Autodesk Inventor part; units mm, degrees
ref_plane "YZ Plane" through (0, 0, 0) normal (1, 0, 0) x (0, 1, 0)
ref_plane "XZ Plane" through (0, 0, 0) normal (0, 1, 0) x (-1, 0, 0)
ref_plane "XY Plane" through (0, 0, 0) normal (0, 0, 1) x (1, 0, 0)
sketch "Sketch2" plane through (0, 0, 0) normal (0, 0, 1) x (1, 0, 0)
  line L0 (0, 12.7) -> (3.6703, 12.7)
  line L1 (0, 12.7) -> (-3.6703, 12.7)
  line L2 (0, 0) -> (3.6703, 0)
  line L3 (0, 0) -> (-3.6703, 0)
  line L4 (-3.6703, 0) -> (-7.3406, 6.35)
  line L5 (-7.3406, 6.35) -> (-3.6703, 12.7)
  line L6 (3.6703, 12.7) -> (7.3406, 6.35)
  line L7 (7.3406, 6.35) -> (3.6703, 0)
  line L8 (0, 0) -> (0, 6.35)
  circle A0 centre (0, 6.35) radius 8.255
  dimension "d11" = 6.35
  dimension "d12" = 16.51
extrude "Extrusion2" add sketch "Sketch2" along normal blind 6.223
sketch "Sketch3" plane through (0, 6.35, 6.223) normal (0, 0, 1) x (1, 0, 0)
  line L0 (-3.6703, -6.35) -> (-7.3406, 0)
  line L1 (-7.3406, 0) -> (-3.6703, 6.35)
  line L2 (-3.6703, 6.35) -> (3.6703, 6.35)
  line L3 (3.6703, 6.35) -> (7.3406, 0)
  line L4 (7.3406, 0) -> (3.6703, -6.35)
  line L5 (3.6703, -6.35) -> (-3.6703, -6.35)
  circle A0 centre (0, 0) radius 8.255
  point P0 (0, -6.35)
extrude "Extrusion3" add sketch "Sketch3" along normal blind 3.302
sketch "Sketch4" plane through (0, 6.35, 9.525) normal (0, 0, 1) x (1, 0, 0)
  line L0 (-7.3406, 0) -> (-3.6703, 6.35)
  line L1 (-3.6703, 6.35) -> (3.6703, 6.35)
  line L2 (3.6703, 6.35) -> (7.3406, 0)
  line L3 (7.3406, 0) -> (3.6703, -6.35)
  line L4 (3.6703, -6.35) -> (-3.6703, -6.35)
  line L5 (-3.6703, -6.35) -> (-7.3406, 0)
  circle A0 centre (0, 0) radius 8.255
  point P0 (0, -6.35)
extrude "Extrusion4" add sketch "Sketch4" along normal blind 6.5786
sketch "Sketch5" plane through (0, 6.35, 16.1036) normal (0, 0, 1) x (1, 0, 0)
  line L0 (-16.3467, 15.7745) -> (15.1254, 15.7745)
  line L1 (15.1254, 15.7745) -> (15.1254, -12.8793)
  line L2 (15.1254, -12.8793) -> (-16.3467, -12.8793)
  line L3 (-16.3467, -12.8793) -> (-16.3467, 15.7745)
  point P0 (0, -6.35)
extrude "Extrusion5" cut sketch "Sketch5" against normal blind 6.5786
sketch "Sketch8" plane through (0, 6.35, 9.525) normal (0, 0, 1) x (1, 0, 0)
  line L0 (-7.3406, 0) -> (-3.6703, -6.35)
  line L1 (-3.6703, 6.35) -> (-7.3406, 0)
  line L2 (3.6703, 6.35) -> (-3.6703, 6.35)
  line L3 (7.3406, 0) -> (3.6703, 6.35)
  line L4 (3.6703, -6.35) -> (7.3406, 0)
  line L5 (-3.6703, -6.35) -> (3.6703, -6.35)
  circle A0 centre (0, 0) radius 8.255
  point P0 (0, -6.35)
extrude "Extrusion7" add sketch "Sketch8" along normal blind 15.875
sketch "Sketch9" plane through (0, 6.35, 25.4) normal (0, 0, 1) x (1, 0, 0)
  line L0 (-7.3406, 0) -> (-3.6703, 6.35)
  line L1 (-3.6703, 6.35) -> (3.6703, 6.35)
  line L2 (3.6703, 6.35) -> (7.3406, 0)
  line L3 (7.3406, 0) -> (3.6703, -6.35)
  line L4 (3.6703, -6.35) -> (-3.6703, -6.35)
  line L5 (-3.6703, -6.35) -> (-7.3406, 0)
  circle A0 centre (0, 0) radius 8.255
  point P0 (0, -6.35)
extrude "Extrusion8" cut sketch "Sketch9" against normal blind 21.7424
sketch "Sketch10" plane through (0, 6.35, 3.6576) normal (0, 0, 1) x (1, 0, 0)
  line L0 (-7.3406, 0) -> (-3.6703, -6.35)
  line L1 (-3.6703, 6.35) -> (-7.3406, 0)
  line L2 (3.6703, 6.35) -> (-3.6703, 6.35)
  line L3 (7.3406, 0) -> (3.6703, 6.35)
  line L4 (3.6703, -6.35) -> (7.3406, 0)
  line L5 (-3.6703, -6.35) -> (3.6703, -6.35)
  circle A0 centre (0, 0) radius 8.255
  point P0 (0, -6.35)
extrude "Extrusion9" add sketch "Sketch10" along normal blind 9.1948
sketch "Sketch11" plane through (0, 6.35, 12.8524) normal (0, 0, 1) x (1, 0, 0)
  line L0 (-15.4934, 11.3446) -> (16.2643, 11.3446)
  line L1 (16.2643, 11.3446) -> (16.2643, -11.0726)
  line L2 (16.2643, -11.0726) -> (-15.4934, -11.0726)
  line L3 (-15.4934, -11.0726) -> (-15.4934, 11.3446)
  point P0 (0, -6.35)
extrude "Extrusion10" cut sketch "Sketch11" against normal blind 1.651
properties part number ".441Spacer"
The listing builds one solid part. Answer for the finished solid, in the listing's coordinates (mm). A direction names the side the tool comes from. Coordinates: 2 decimals unless noted, no trailing zeros. Loops run counter-clockwise (first coordinate to the right, second up) from the corner with the lowest first, then second, coordinate; pieces in that order, holes last. Notation, with made-up numbers: M -33.75,14 L 1.25,14 A34 cw 1.25,49 Z; hole C 86,76.5 d9. An arc over 180 degrees is marked long. Answer as a JSON object with one key per item and string values. Group by question number.
Item 1: Consider L1, parallel to X at y = 4.25, z = 10; L2, parallel to X at y = 3.5, z = 8; L3, parallel to Y at x = 3.75, z = 1.5. Determine where each line is inside the solid, lowest interval first.
Item 2: Section D-D (y = 13) is taken. Write down the section's boundary in (x, z), and give its area (3 significant figures).
Item 3: Section A-A (x = 0) is taken. Write down the section's boundary in (y, z) (3 decimals), and give its area (3 significant figures).
Item 4: Each of these flat-tipped pins is pushed along its axis until it touches: P1, Ø5, axis at y = 3.5, z = 10, coming from the +X side; P2, Ø5, axis at x = -4, z = 3, coming from the +Y side; P3, Ø4, axis at y = 9.5, z = 7, coming from the -X side. Where does it stop, or does it pass through?
Item 5: Section C-C (y = 8.75) is taken. Write down the section's boundary in (x, z).
Item 6: Section B-B (z = 3) is taken. Write down the section's boundary in (x, y) (3 decimals).
Item 7: Which of the six approach directions +Z, -Z, +X, -X, +Y, -Y give full straight-line access (tool end or side, diameter ignored) to faces 5 (the face through (0, 12.7, 6)), 6 (the face through (-5, 2, 0))?
Item 8: Determine the mould class of faces 1 (the face through (-5, 2, 11.201)), 2 (the face through (5.53, 9.48, 5.52)), 3 (the face through (-1.79, 14.41, 5.52)), 4 (the face through (-5.53, 3.22, 5.52)) for opening direction Y: +Y half, -Y half, draft (parallel to the pull), parting line (faces both ways), or undercut.
Solved:
{
 "1": {"L1": "x = -7.98 to -6.13, 6.13 to 7.98", "L2": "x = -7.75 to -5.69, 5.69 to 7.75", "L3": "y = -1 to 0.14, 12.56 to 13.7"},
 "2": {"outline": "M -4.89,0 L 4.89,0 L 4.89,11.2 L -4.89,11.2 Z", "area": "110 mm2"},
 "3": {"outline": "M -1.905,0 L 0,0 L 0,11.201 L -1.905,11.201 Z; M 12.7,0 L 14.605,0 L 14.605,11.201 L 12.7,11.201 Z", "area": "42.7 mm2"},
 "4": {"P1": "stops at x = 8.25", "P2": "stops at y = 14.47", "P3": "stops at x = -8.17"},
 "5": {"outline": "M -7.9,0 L -5.95,0 L -5.95,11.2 L -7.9,11.2 Z; M 5.95,0 L 7.9,0 L 7.9,11.2 L 5.95,11.2 Z"},
 "6": {"outline": "C 0,6.35 d16.51; hole M -7.341,6.35 L -3.67,0 L 3.67,0 L 7.341,6.35 L 3.67,12.7 L -3.67,12.7 Z"},
 "7": {"face 5": "+Z, -Z", "face 6": "-Z, +X, -X, +Y, -Y"},
 "8": {"face 1": "draft", "face 2": "undercut", "face 3": "parting line", "face 4": "undercut"}
}
